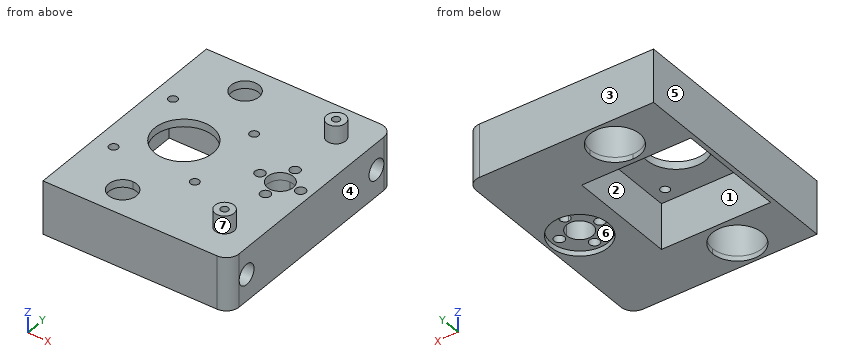
from build123d import *

# Parameters (mm, degrees)
F1_DEPTH  = 2
F2_R      = 9.75
F2_W      = 43
F2_H      = 43
F2_R_2    = 11.25
F2_R_3    = 2
F3_DEPTH  = 16
F4_R      = 9.75
F4_R_2    = 2
F4_W      = 43
F4_H      = 43
F4_R_3    = 5.1
F4_R_4    = 1.75
F4_R_5    = 11.5
F5_DEPTH  = 3
F7_DEPTH  = 40
F6_R      = 4
F8_DEPTH  = 35
F9_R      = 3.75
F9_R_2    = 1.5
F10_DEPTH = 7


# Not quite as in the source:
# - after a boolean that leaves OpenCascade's solid faulty, fix() repairs it
# - a feature names something its author has since deleted; it is built from what else it names


with BuildPart() as f1:
    # F0 (on Top) → F1 (new body)
    with BuildSketch(Plane.XY):
        with BuildLine():
            Line((45.2909459174, 44.0599285066), (23.2912804931, 44.0599285066))
            Line((23.2912804931, 44.0599285066), (-23.2912804931, 44.0599285066))
            Line((-23.2912804931, 44.0599285066), (-23.2912804931, -44.0599285066))
            Line((-23.2912804931, -44.0599285066), (23.2912804931, -44.0599285066))
            Line((23.2912804931, -44.0599285066), (45.2909459174, -44.0599285066))
            ThreePointArc((45.2909459174, -44.0599285066), (48.8264798233, -42.5954624125), (50.2909459174, -39.0599285066))
            Line((50.2909459174, -39.0599285066), (50.2909459174, -23.5600714934))
            Line((50.2909459174, -23.5600714934), (50.2909459174, 23.5599285066))
            Line((50.2909459174, 23.5599285066), (50.2909459174, 39.0599285066))
            ThreePointArc((50.2909459174, 39.0599285066), (48.8264798233, 42.5954624125), (45.2909459174, 44.0599285066))
        make_face()
        with BuildLine():
            ThreePointArc((9.75, -33), (-6.8942911166, -39.8942911166), (0, -23.25))
            ThreePointArc((0, -23.25), (6.8942911166, -26.1057088834), (9.75, -33))
        make_face(mode=Mode.SUBTRACT)
        Polygon((21.5, 21.5), (21.5, 0), (21.5, -21.5), (0, -21.5), (-21.5, -21.5), (-21.5, 21.5), (0, 21.5), (21.4772019535, 21.5), align=None, mode=Mode.SUBTRACT)
        with BuildLine():
            ThreePointArc((9.75, 33), (6.8942911166, 26.1057088834), (0, 23.25))
            ThreePointArc((0, 23.25), (-6.8942911166, 39.8942911166), (9.75, 33))
        make_face(mode=Mode.SUBTRACT)
        with BuildLine():
            ThreePointArc((26.75, 0), (38, 11.25), (49.25, 0))
            ThreePointArc((49.25, 0), (38, -11.25), (26.75, 0))
        make_face(mode=Mode.SUBTRACT)
    extrude(amount=F1_DEPTH)

    # F2 (on face) → F3 (join)
    with BuildSketch(Plane.XY.offset(2)):
        with BuildLine():
            ThreePointArc((50.2909459174, 39.0599285066), (48.8264798233, 42.5954624125), (45.2909459174, 44.0599285066))
            Line((45.2909459174, 44.0599285066), (-23.2912804931, 44.0599285066))
            Line((-23.2912804931, 44.0599285066), (-23.2912804931, -44.0599285066))
            Line((-23.2912804931, -44.0599285066), (45.2909459174, -44.0599285066))
            ThreePointArc((45.2909459174, -44.0599285066), (48.8264798233, -42.5954624125), (50.2909459174, -39.0599285066))
            Line((50.2909459174, -39.0599285066), (50.2909459174, 39.0599285066))
        make_face()
        with Locations((0, -33)):
            Circle(F2_R, mode=Mode.SUBTRACT)
        Rectangle(F2_W, F2_H, mode=Mode.SUBTRACT)
        with Locations((0, 33)):
            Circle(F2_R, mode=Mode.SUBTRACT)
        with Locations((38, 0)):
            Circle(F2_R_2, mode=Mode.SUBTRACT)
        with Locations((38, 0)):
            Circle(F2_R_2)
        with Locations((38, -8)):
            Circle(F2_R_3, mode=Mode.SUBTRACT)
        with Locations((30, 0)):
            Circle(F2_R_3, mode=Mode.SUBTRACT)
        with BuildLine():
            ThreePointArc((38, 5.1), (41.6062445841, 3.6062445841), (43.1, 0))
            ThreePointArc((43.1, 0), (34.3937554159, -3.6062445841), (38, 5.1))
        make_face(mode=Mode.SUBTRACT)
        with BuildLine():
            ThreePointArc((40, 8), (39.4142135624, 6.5857864376), (38, 6))
            ThreePointArc((38, 6), (36.5857864376, 9.4142135624), (40, 8))
        make_face(mode=Mode.SUBTRACT)
        with BuildLine():
            ThreePointArc((48, 0), (46, -2), (44, 0))
            ThreePointArc((44, 0), (46, 2), (48, 0))
        make_face(mode=Mode.SUBTRACT)
    extrude(amount=F3_DEPTH)

    # F4 (on face) → F5 (join)
    with BuildSketch(Plane.XY.offset(18)):
        with BuildLine():
            Line((50.2909459174, -39.0599285066), (50.2909459174, 39.0599285066))
            ThreePointArc((50.2909459174, 39.0599285066), (48.8264798233, 42.5954624125), (45.2909459174, 44.0599285066))
            Line((45.2909459174, 44.0599285066), (-23.2912804931, 44.0599285066))
            Line((-23.2912804931, 44.0599285066), (-23.2912804931, -44.0599285066))
            Line((-23.2912804931, -44.0599285066), (45.2909459174, -44.0599285066))
            ThreePointArc((45.2909459174, -44.0599285066), (48.8264798233, -42.5954624125), (50.2909459174, -39.0599285066))
        make_face()
        with Locations((0, -33)):
            Circle(F4_R, mode=Mode.SUBTRACT)
        with Locations((38, -8)):
            Circle(F4_R_2, mode=Mode.SUBTRACT)
        Rectangle(F4_W, F4_H, mode=Mode.SUBTRACT)
        with Locations((0, 33)):
            Circle(F4_R, mode=Mode.SUBTRACT)
        with Locations((30, 0)):
            Circle(F4_R_2, mode=Mode.SUBTRACT)
        with Locations((38, 0)):
            Circle(F4_R_3, mode=Mode.SUBTRACT)
        with Locations((38, 8)):
            Circle(F4_R_2, mode=Mode.SUBTRACT)
        with Locations((46, 0)):
            Circle(F4_R_2, mode=Mode.SUBTRACT)
        Rectangle(F4_W, F4_H)
        with Locations((-16, -16)):
            Circle(F4_R_4, mode=Mode.SUBTRACT)
        with Locations((16, -16)):
            Circle(F4_R_4, mode=Mode.SUBTRACT)
        with Locations((-16, 16)):
            Circle(F4_R_4, mode=Mode.SUBTRACT)
        Circle(F4_R_5, mode=Mode.SUBTRACT)
        with Locations((16, 16)):
            Circle(F4_R_4, mode=Mode.SUBTRACT)
        with Locations((0, -33)):
            Circle(F4_R)
        with Locations((0, 33)):
            Circle(F4_R)
    extrude(amount=F5_DEPTH)

    # F0 (on Top) → F7 (cut)
    with BuildSketch(Plane.XY):
        with BuildLine():
            ThreePointArc((5.5, -33), (3.8890872965, -29.1109127035), (0, -27.5))
            ThreePointArc((0, -27.5), (-3.8890872965, -36.8890872965), (5.5, -33))
        make_face()
        with BuildLine():
            ThreePointArc((5.5, 33), (-3.8890872965, 36.8890872965), (0, 27.5))
            ThreePointArc((0, 27.5), (3.8890872965, 29.1109127035), (5.5, 33))
        make_face()
    extrude(amount=F7_DEPTH, mode=Mode.SUBTRACT)

    add(f1.part.fix(), mode=Mode.REPLACE)

    # F6 (on face) → F8 (cut)
    with BuildSketch(Plane.YZ.offset(50.2909459174)):
        with Locations((35, 10.5)):
            Circle(F6_R)
        with Locations((-35, 10.5)):
            Circle(F6_R)
    extrude(amount=-F8_DEPTH, mode=Mode.SUBTRACT)

    # F9 (on face) → F10 (join)
    with BuildSketch(Plane.XY.offset(21)):
        with Locations((37.9999959174, 30.0599285066)):
            Circle(F9_R)
        with Locations((37.9999959174, 30.0599285066)):
            Circle(F9_R_2, mode=Mode.SUBTRACT)
        with Locations((37.9999959174, -30.0599285066)):
            Circle(F9_R)
        with Locations((37.9999959174, -30.0599285066)):
            Circle(F9_R_2, mode=Mode.SUBTRACT)
    extrude(amount=F10_DEPTH)


solid = f1.part
Model file for the job. Use its own axes, mm. Face numbers are marked on the shaded views. A direction names the side the tool comes from. Give positions to 0.01 mm unless a question says otherwise; leave off trailing zeros. Order: outer loops, then holes, each group sorted by start corner. A loop starts at its lowest first (then second) coordinate and runs counter-clockwise, first axis right, second up. Notation, with made-up numbers: (-28, 30) -> (-6, 30) arc R8 cw to (-6, 42) -> close; hole circle Ø5 at (82, -25.75). An arc over 180 degrees is marked (long way). Use CSV: the item, a comma, the result in double quotes.
1. Band-saw the part on C-C, the plane y = 35. Give the cut face in (x, z).
Outcome:
outline,"(-23.29, 0) -> (-9.54, 0) -> (-9.54, 18) -> (-5.12, 18) -> (-5.12, 21) -> (-23.29, 21) -> close; (5.12, 18) -> (9.54, 18) -> (9.54, 0) -> (50.29, 0) -> (50.29, 6.5) -> (15.29, 6.5) -> (15.29, 14.5) -> (50.29, 14.5) -> (50.29, 21) -> (5.12, 21) -> close"
2. Drop flat-ended pins along their axis: pin 1 (11.5 mm diameter, centred on x = 0, y = -33, fed in from +Z); pin 2 (17.5 mm diameter, centred on x = 0, y = 33, fed in from -Z); pin 3 (10 mm diameter, centred on x = 0, y = -33, fed in from -Z). Give the stop position or say it passes through.
Outcome:
pin 1,"z = 21"
pin 2,"z = 18"
pin 3,"through"
3. Band-saw the part on A-A, the plane z = 10.5. Count the separate pieces of the cut face and the enclosed holes in it, then the cut area to 3 significant figures.
Outcome:
separate pieces,"1"
enclosed holes,"8"
area,"3,340 mm²"
4. Band-saw the part on B-B, the plane x = 30. Give the cut face in (y, z), then the cut area to 3 significant figures.
Outcome:
outline,"(-44.06, 0) -> (-7.91, 0) -> (-7.91, 2) -> (-2, 2) -> (-2, 21) -> (-44.06, 21) -> close; (2, 2) -> (7.91, 2) -> (7.91, 0) -> (44.06, 0) -> (44.06, 21) -> (2, 21) -> close; hole circle Ø8 at (-35, 10.5); hole circle Ø8 at (35, 10.5)"
area,"1,640 mm²"
5. Mould opens along Y. For the marked faces 1, 2, 3 and 4 say: +Y half, -Y half, draft (parallel to the pull), parting line (faces both ways), or undercut.
Outcome:
face 1,"undercut"
face 2,"undercut"
face 3,"+Y half"
face 4,"draft"
6. 3-axis set-ups, long thin cutter, end or side, ignore diameter. For the marked faces 5, 6 and 7: which of +Z, -Z, +X, -X, +Y, -Y reach the whole face in a straight line?
Outcome:
face 5,"+Z, -Z, -X, +Y, -Y"
face 6,"-Z"
face 7,"+Z"
7. Drill centre lines: line 1 along Y through (x, z) = (-16, 19.7); line 2 along Y through (x, z) = (30, 10.25); line 3 along Y through (x, z) = (14, 7). Where is each one in solid material? Low to high. Write a range as from..to.
Outcome:
line 1,"-44.06..-17.75, -14.25..14.25, 17.75..44.06"
line 2,"-44.06..-38.99, -31.01..-2, 2..31.01, 38.99..44.06"
line 3,"-44.06..-21.5, 21.5..44.06"
8. Band-saw the part on D-D, the plane x = 19.5. Give the cut face in (y, z).
Outcome:
outline,"(-44.06, 0) -> (-21.5, 0) -> (-21.5, 18) -> (21.5, 18) -> (21.5, 0) -> (44.06, 0) -> (44.06, 21) -> (-44.06, 21) -> close; hole circle Ø8 at (-35, 10.5); hole circle Ø8 at (35, 10.5)"
